```python
from build123d import *

# Parameters (mm, degrees)
SKETCH1_R           = 1.5
BOSS_EXTRUDE1_DEPTH = 1
BOSS_EXTRUDE2_DEPTH = 5


with BuildPart() as part:
    # Sketch1 → Boss-Extrude1 (new body)
    with BuildSketch(Plane(origin=(0, 0, 0), x_dir=(1, 0, 0), z_dir=(0, 1, 0))):
        with BuildLine():
            Line((-4.65, -9), (4.65, -9))
            ThreePointArc((4.65, -9), (7.725914498, -7.725914498), (9, -4.65))
            Line((9, -4.65), (9, 4.65))
            ThreePointArc((9, 4.65), (7.725914498, 7.725914498), (4.65, 9))
            Line((4.65, 9), (-4.65, 9))
            ThreePointArc((-4.65, 9), (-7.725914498, 7.725914498), (-9, 4.65))
            Line((-9, 4.65), (-9, -4.65))
            ThreePointArc((-9, -4.65), (-7.725914498, -7.725914498), (-4.65, -9))
        make_face()
        Circle(SKETCH1_R, mode=Mode.SUBTRACT)
    extrude(amount=BOSS_EXTRUDE1_DEPTH)

    # Sketch2 → Boss-Extrude2 (add)
    with BuildSketch(Plane(origin=(0, 1, 0), x_dir=(1, 0, 0), z_dir=(0, 1, 0))):
        Polygon((-8, 4.65), (-4.65, 8), (4.65, 8), (8, 4.65), (8, -4.65), (4.65, -8), (-4.65, -8), (-8, -4.65), align=None)
        Polygon((-7, 4.235786438), (-4.235786438, 7), (4.235786438, 7), (7, 4.235786438), (7, -4.235786438), (4.235786438, -7), (-4.235786438, -7), (-7, -4.235786438), align=None, mode=Mode.SUBTRACT)
    extrude(amount=BOSS_EXTRUDE2_DEPTH)


solid = part.part
```
Model file for the job. Use its own axes, mm. A direction names the side the tool comes from. Give positions to 0.01 mm unless a question says otherwise; leave off trailing zeros. Loops run counter-clockwise (first coordinate to the right, second up) from the corner with the lowest first, then second, coordinate; pieces in that order, holes last. Notation, with made-up numbers: (25.5, 43.25) -> (81.5, 43.25) arc R4 ccw to (81.5, 50.25) -> close; hole circle Ø5 at (21, 52.5). An arc over 180 degrees is marked (long way). Write each question's results on one line, items separated by ' | '.
(1) Tool access for faces 5 (the flat face through (0, 3, 8)), 6 (the flat face through (-5.637, 3.465, -5.599)), 7 (the flat face through (6.3, 3.46, -6.35)): list every direction of +Z, -Z, +X, -X, +Y, -Y with a clear straight run to the whole face (end or side of a thin tool).
Geometry results:
face 5: +Z, +X, -X, +Y | face 6: +Y | face 7: -Z, +X, +Y
(2) Cut at A-A on z = 0. List the corners of the cut face in (x, y), and give its area (3 significant figures).
Geometry results:
outline: (-9, 0) -> (-1.5, 0) -> (-1.5, 1) -> (-7, 1) -> (-7, 6) -> (-8, 6) -> (-8, 1) -> (-9, 1) -> close; (1.5, 0) -> (9, 0) -> (9, 1) -> (8, 1) -> (8, 6) -> (7, 6) -> (7, 1) -> (1.5, 1) -> close | area: 25.0 mm²
(3) Flat gauge pins, fed straight in: pin 1 Ø1.5 at (y, z) = (2.5, -1.5) entering from +X; pin 2 Ø5 at (x, z) = (1.5, 2) entering from +Y; pin 3 Ø1.5 at (x, y) = (1, 4.5) entering from +Z; pin 4 Ø8 at (x, z) = (-2.5, -4) entering from +Y. Where does each tip first touch, or does it go through?
Geometry results:
pin 1: stops at x = 8 | pin 2: stops at y = 1 | pin 3: stops at z = 8 | pin 4: stops at y = 6
(4) Pull direction Z, two halves, no side cores. Call faces 1 (the flat face through (-8, 3, 0)), 2 (the flat face through (6.35, 3.46, 6.3)), 3 (the flat face through (-6.35, 3.46, -6.3)), 4 (the flat face through (0, 3, 7)): released by +Z, released by -Z, zero draft, split by the parting line, or undercut.
Geometry results:
face 1: zero draft | face 2: released by +Z | face 3: released by -Z | face 4: undercut
(5) Cut at C-C on y = 2.7. List the corners of the cut face in (x, z).
Geometry results:
outline: (-8, -4.65) -> (-4.65, -8) -> (4.65, -8) -> (8, -4.65) -> (8, 4.65) -> (4.65, 8) -> (-4.65, 8) -> (-8, 4.65) -> close; hole (-7, -4.24) -> (-4.24, -7) -> (4.24, -7) -> (7, -4.24) -> (7, 4.24) -> (4.24, 7) -> (-4.24, 7) -> (-7, 4.24) -> close
(6) Cut at B-B on x = 0. List the corners of the cut face in (y, z).
Geometry results:
outline: (0, -9) -> (1, -9) -> (1, -8) -> (6, -8) -> (6, -7) -> (1, -7) -> (1, -1.5) -> (0, -1.5) -> close; (0, 1.5) -> (1, 1.5) -> (1, 7) -> (6, 7) -> (6, 8) -> (1, 8) -> (1, 9) -> (0, 9) -> close
(7) Cut at D-D on x = 4. List the corners of the cut face in (y, z), and give its area (3 significant figures).
Geometry results:
outline: (0, -9) -> (1, -9) -> (1, -8) -> (6, -8) -> (6, -7) -> (1, -7) -> (1, 7) -> (6, 7) -> (6, 8) -> (1, 8) -> (1, 9) -> (0, 9) -> close | area: 28.0 mm²
(8) Probe line 1 along Z through (x, y) = (2.25, 5.55); line 2 along X through (y, z) = (0.6, 0). List the from-to ranges inside material, lowest first.
Geometry results:
line 1: z = -8 to -7, 7 to 8 | line 2: x = -9 to -1.5, 1.5 to 9
